Read the model definition and answer for the solid it produces. Units are mm, in the model's axes. A direction names the side the tool comes from. Coordinates: 2 decimals unless noted, no trailing zeros. Write each loop counter-clockwise with the first axis right and the second up, starting at its lowest first coordinate (ties: lowest second). Pieces come first, ordered by that corner, then holes.
(1) The mould has two halves that part along Z. Classify faces 1 (the cylindrical face through (14.2, -1.44, -0.7)), 2 (the cylindrical face through (15.28, -3.81, -1.22)), 3 (the flat face through (26, -0.9, 3)): +Z half, -Z half, draft (parallel to the pull), parting line (faces both ways), or undercut.
(2) Section A-A on x = 16 is taken. Write down the section's boundary in (y, z).
(3) Find the intervals of material crossed by probe 1 along Y at (x, z) = (24, 0); probe 2 along Y at (x, z) = (13.5, 0); probe 3 along Z at (x, y) = (36.5, -1), in increasing order.
(4) Which of the six approach directions +Z, -Z, +X, -X, +Y, -Y give full straight-line access (tool end or side, diameter ignored) to faces 4 (the flat face through (7, 1, 3)), 5 (the flat face through (36.49, -2.08, -0.05)), 6 (the flat face through (7, -1, 3)), 7 (the flat face through (0, 0, -2)), 8 (the flat face through (26, -0.9, -3))?
(5) Section D-D on z = -2.5 is taken. Write down the section's boundary in (x, y).
(6) Given pin 1 (1.5 mm diameter, centred on y = -2, z = 0.5, fed in from +X); pin 2 (4 mm diameter, centred on x = 30.5, y = -3, fed in from +Z); pin 3 (0.8 mm diameter, centred on x = 8, z = 3, fed in from -Y); pin 4 (1.5 mm diameter, centred on y = 1, z = 1.5, fed in from -X), each flat-ended and moving along its own axis, determine where each tip first touches the part or whether it passes through.
(7) Section C-C on y = 0 is taken. Write down the section's boundary in (x, z), then the cut area to 3 significant figures.
(8) Section B-B on z = 1.75 is taken. Write down the section's boundary in (x, y), then the cut area to 3 significant figures.
Autodesk Inventor part; units mm, degrees
ref_plane "YZ Plane" through (0, 0, 0) normal (1, 0, 0) x (0, 1, 0)
ref_plane "XZ Plane" through (0, 0, 0) normal (0, 1, 0) x (-1, 0, 0)
ref_plane "XY Plane" through (0, 0, 0) normal (0, 0, 1) x (1, 0, 0)
sketch "Sketch1" plane through (0, 0, 0) normal (1, 0, 0) x (0, 1, 0)
  circle A0 centre (0, 0) radius 4
  dimension "d0" = 8
extrude "Extrusion1" add sketch "Sketch1" along normal blind 40
sketch "Sketch2" plane through (40, 0, 0) normal (1, 0, 0) x (0, 0, -1)
  line L0 (-4, 2.5) -> (4, 2.5)
  line L1 (4, 2.5) -> (4, -0.9)
  line L2 (4, -0.9) -> (-4, -0.9)
  line L3 (-4, -0.9) -> (-4, 2.5)
  point P0 (0, 0)
  dimension "d3" = 8
  dimension "d4" = 3.4
  dimension "d5" = 2.5
  dimension "d6" = 4
extrude "Extrusion2" cut sketch "Sketch2" against normal blind 25
sketch "Sketch3" plane through (0, 0, 0) normal (-1, 0, 0) x (0, 0, 1)
  circle A0 centre (0, 0) radius 1.6
  dimension "d9" = 3.2
extrude "Extrusion3" cut sketch "Sketch3" against normal through all
sketch "Sketch4" plane through (0, 0, 0) normal (0, 0, 1) x (1, 0, 0)
  line L0 (40, 2.5) -> (40, 4)
  line L1 (40, 4) -> (35.3812, -4)
  line L2 (0, -4) -> (40, -4)
  line L3 (40, 4) -> (49.2376, 4) construction
  line L4 (35.3812, -4) -> (40, -4)
  line L5 (40, 4) -> (40, -4)
  point P0 (0, 0)
  dimension "d12" = 120
extrude "Extrusion4" cut sketch "Sketch4" along normal through all both and the other way through all
sketch "Sketch6" plane through (0, 0, 0) normal (-1, 0, 0) x (0, 0, 1)
  line L0 (4, 1) -> (1.2, 1)
  line L1 (1.2, 1) -> (1.2, -1)
  line L2 (1.2, -1) -> (4, -1)
  line L3 (4, -1) -> (4, 1)
  point P0 (0, 0)
  dimension "d23" = 2
  dimension "d24" = 4
  dimension "d25" = 1
  dimension "d27" = 1.2
extrude "Extrusion6" cut sketch "Sketch6" against normal up to surface (15 mm away)
properties part number "Main_tip_coupler"
Response:
1. face 1: undercut
1. face 2: parting line
1. face 3: draft
2. outline: (-0.9, -3.9) - (-0.9, -1.32) arc R1.6 cw to (-0.9, 1.32) - (-0.9, 3.9) arc R4 ccw to start; (2.5, -3.12) arc R4 ccw to (2.5, 3.12) - close
3. probe 1: y = -4 to -1.6, 2.5 to 4
3. probe 2: y = -4 to -1.6, 1.6 to 4
3. probe 3: z = -3.87 to -1.25, 1.25 to 3.87
4. face 4: +Z, +X, -X
4. face 5: +Z, -Z, +X, -Y
4. face 6: +Z, -X
4. face 7: +Z, -Z, -X, +Y, -Y
4. face 8: +Z, -Z, +X
5. outline: (0, -3.12) - (35.89, -3.12) - (37.17, -0.9) - (15, -0.9) - (15, 2.5) - (39.13, 2.5) - (39.49, 3.12) - (0, 3.12) - close
6. pin 1: stops at x = 36.91
6. pin 2: stops at z = 3.87
6. pin 3: stops at y = -3.04
6. pin 4: stops at x = 0
7. outline: (0, -4) - (15, -4) - (15, -1.6) - (0, -1.6) - close
7. area: 36.0 mm2
8. outline: (0, -3.6) - (35.61, -3.6) - (37.17, -0.9) - (15, -0.9) - (15, -1) - (0, -1) - close; (0, 1) - (15, 1) - (15, 2.5) - (39.13, 2.5) - (39.77, 3.6) - (0, 3.6) - close
8. area: 162 mm2
